from build123d import *

# Parameters (mm, degrees)
SKETCH1_R           = 11.1252
BOSS_EXTRUDE1_DEPTH = 12.7
SKETCH4_R           = 8.255
CUT_EXTRUDE2_DEPTH  = 10
CUT_EXTRUDE1_DEPTH  = 28.930993094
CUT_EXTRUDE3_REACH  = 28.204
SKETCH5_R           = 1.2065


with BuildPart() as part:
    # Sketch1 → Boss-Extrude1 (new body)
    with BuildSketch(Plane(origin=(0, 0, 0), x_dir=(1, 0, 0), z_dir=(0, 1, 0))):
        with Locations(Location((0, 0, 0), (0, 0, 270))):
            Circle(SKETCH1_R)
    extrude(amount=BOSS_EXTRUDE1_DEPTH)

    # Sketch4 → Cut-Extrude2 (cut)
    with BuildSketch(Plane(origin=(0, 12.7, 0), x_dir=(1, 0, 0), z_dir=(0, 1, 0))):
        with Locations(Location((0, 0, 0), (0, 0, 270))):
            Circle(SKETCH4_R)
    extrude(amount=-CUT_EXTRUDE2_DEPTH, mode=Mode.SUBTRACT)

    # Sketch3 → Cut-Extrude1 (cut, through all)
    with BuildSketch(Plane(origin=(0, 0, -11.1252), x_dir=(-1, 0, 0), z_dir=(0, 0, -1))):
        with BuildLine():
            Line((-1.905, 12.7), (-1.905, 4.605))
            ThreePointArc((-1.905, 4.605), (0, 2.7), (1.905, 4.605))
            Line((1.905, 4.605), (1.905, 12.7))
            Line((1.905, 12.7), (-1.905, 12.7))
        make_face()
    extrude(amount=-CUT_EXTRUDE1_DEPTH, mode=Mode.SUBTRACT)

    # Sketch2 → Revolve3 (revolve)
    with BuildSketch(Plane.XY):
        with BuildLine():
            Line((0, 20.955), (0, 1.905))
            ThreePointArc((0, 1.905), (9.525, 11.43), (0, 20.955))
        make_face()
    revolve(axis=Axis((0, 20.955, 0), (0, -1, 0)))

    # Sketch5 → Cut-Extrude3 (cut, up to next)
    with BuildSketch(Plane.XZ, mode=Mode.PRIVATE) as cut_extrude3_sk1:
        with Locations(Location((0, 7.747, 0), (0, 0, 270))):
            Circle(SKETCH5_R)
    cut_extrude3_tool1 = extrude(cut_extrude3_sk1.sketch, amount=-CUT_EXTRUDE3_REACH, mode=Mode.PRIVATE) & part.part
    # Sketch5 → Cut-Extrude3 (cut, up to next)
    with BuildSketch(Plane.XZ, mode=Mode.PRIVATE) as cut_extrude3_sk2:
        with Locations(Location((0, -7.747, 0), (0, 0, 270))):
            Circle(SKETCH5_R)
    cut_extrude3_tool2 = extrude(cut_extrude3_sk2.sketch, amount=-CUT_EXTRUDE3_REACH, mode=Mode.PRIVATE) & part.part
    add(cut_extrude3_tool1.solids().sort_by_distance((0, 0, 7.747))[0], mode=Mode.SUBTRACT)
    add(cut_extrude3_tool2.solids().sort_by_distance((0, 0, -7.747))[0], mode=Mode.SUBTRACT)


solid = part.part
Design review of the part built by this model. Coordinates are the model's own, in mm. A direction names the side the tool comes from. Coordinates: 2 decimals unless noted, no trailing zeros. Order: outer loops, then holes, each group sorted by start corner. A loop starts at its lowest first (then second) coordinate and runs counter-clockwise, first axis right, second up. Notation, with made-up numbers: (3.5, 83) -> (32.5, 83) arc R33 cw to (32.5, 115) -> close; hole circle Ø6 at (70, -13). An arc over 180 degrees is marked (long way). One line per item, written item: value.
1) We need section C-C, the plane z = -4.25. Give the boundary of the cut face in (x, y), then the cut area to 3 significant figures.
Output values:
outline: (-10.28, 0) -> (10.28, 0) -> (10.28, 12.7) -> (8.43, 12.7) arc R8.52 ccw to (-8.43, 12.7) -> (-10.28, 12.7) -> close; hole (-7.08, 2.7) -> (7.08, 2.7) -> (7.08, 6.68) arc R8.52 cw to (-7.08, 6.68) -> close
area: 335 mm2
2) Clearance check with flat-ended pins moving along their axes: P1, Ø5, axis at x = -2, z = 4, coming from the +Y side; P2, Ø3, axis at x = -8, z = -2, coming from the +Y side; P3, Ø1.5, axis at y = 7, z = 9, coming from the +X side. State where each tip first meets the part, or that it passes through.
Output values:
P1: stops at y = 20.75
P2: stops at y = 18.15
P3: stops at x = 7.46
3) Draft analysis for pull direction Y (two halves, no side actions). For faces 4 (the face through (0.815, 1.513, 8.636)), 5 (the face through (-10, 12.7, -1)), 6 (the face through (-2, 2.7, 4)), state which applies: +Y half, -Y half, draft (parallel to the pull), parting line (faces both ways), or undercut.
Output values:
face 4: draft
face 5: +Y half
face 6: undercut
4) We need section D-D, the plane y = 12. Give the boundary of the cut face in (x, z) (3 decimals).
Output values:
outline: (-1.905, -10.961) -> (-1.905, -9.315) arc R9.508 ccw to (1.905, -9.315) -> (1.905, -10.961) arc R11.125 ccw to (1.905, 10.961) -> (1.905, 9.315) arc R9.508 ccw to (-1.905, 9.315) -> (-1.905, 10.961) arc R11.125 ccw to start
5) We need section A-A, the plane z = 2.5. Give the boundary of the cut face in (x, y), then the cut area to 3 significant figures.
Output values:
outline: (-10.84, 0) -> (10.84, 0) -> (10.84, 12.7) -> (9.1, 12.7) arc R9.19 ccw to (-9.1, 12.7) -> (-10.84, 12.7) -> close; hole (-7.87, 2.7) -> (-2.87, 2.7) arc R9.19 cw to (-7.87, 6.68) -> close; hole (2.87, 2.7) -> (7.87, 2.7) -> (7.87, 6.68) arc R9.19 cw to start
area: 370 mm2
6) Machinability: for faces 1 (the face through (1.905, 8, -10)), 2 (the face through (1.905, 8, 10)), 3 (the face through (-8.253, 4.717, -0.166)), which of the approach directions +Z, -Z, +X, -X, +Y, -Y give a long, thin tool a straight path to every point of the face, cutting with its end or side? Answer none if there is none.
Output values:
face 1: -Z
face 2: +Z
face 3: none
7) To check wall thickness, follow probe 1 along Z at (x, y) = (0, 1.4); probe 2 along Z at (x, y) = (-4.25, 5); probe 3 along Z at (x, y) = (-9, 10.5). State the ranges of each line that lie inside material, in increasing order. Write a range as [from, to].
Output values:
probe 1: z = [-11.13, -8.95], [-6.54, 6.54], [8.95, 11.13]
probe 2: z = [-10.28, -7.08], [-5.6, 5.6], [7.08, 10.28]
probe 3: z = [-6.54, 6.54]
8) We need section B-B, the plane x = 0. Count the separate pieces of the cut face and the enclosed holes in it, then the cut area to 3 significant figures.
Output values:
separate pieces: 3
enclosed holes: 0
area: 328 mm2
